```python
from build123d import *

# Parameters (mm, degrees)
EXTRUDE_1_DEPTH = 1
EXTRUDE_2_DEPTH = 1
EXTRUDE_3_REACH = 17
SKETCH_3_R      = 2.5


with BuildPart() as part:
    # 草图1 → 凸台-拉伸1 (new body)
    with BuildSketch(Plane(origin=(0, 0, 0), x_dir=(1, 0, 0), z_dir=(0, 1, 0))):
        with BuildLine():
            Line((-7, 15), (7, 15))
            ThreePointArc((7, 15), (7.707106781, 14.707106781), (8, 14))
            Line((8, 14), (8, -14))
            ThreePointArc((8, -14), (7.707106781, -14.707106781), (7, -15))
            Line((7, -15), (-7, -15))
            ThreePointArc((-7, -15), (-7.707106781, -14.707106781), (-8, -14))
            Line((-8, -14), (-8, 14))
            ThreePointArc((-8, 14), (-7.707106781, 14.707106781), (-7, 15))
        make_face()
    extrude(amount=EXTRUDE_1_DEPTH)

    # 草图2 → 凸台-拉伸2 (add)
    with BuildSketch(Plane.ZY.offset(8)):
        with BuildLine():
            Line((14, 1), (3.844755362, 32.532743309))
            ThreePointArc((3.844755362, 32.532743309), (-1.048573514, 35.998202631), (-5.749110975, 32.275431702))
            Line((-5.749110975, 32.275431702), (-14, 1))
            Line((-14, 1), (14, 1))
        make_face()
    extrude_2 = extrude(amount=-EXTRUDE_2_DEPTH)

    # 镜向1: 凸台-拉伸2 across plane
    add(extrude_2.mirror(Plane(origin=(0, 0, 0), x_dir=(0, 0, 1), z_dir=(1, 0, 0))))

    # 草图3 → 凸台-拉伸3 (add, up to next)
    with BuildSketch(Plane(origin=(-7, 0, 0), x_dir=(0, 0, -1), z_dir=(1, 0, 0)), mode=Mode.PRIVATE) as extrude_3_sk1:
        with Locations((0.914519578, 31)):
            Circle(SKETCH_3_R)
    extrude_3_tool1 = extrude(extrude_3_sk1.sketch, amount=EXTRUDE_3_REACH, mode=Mode.PRIVATE) - part.part
    add(extrude_3_tool1.solids().sort_by_distance((-7, 31, -0.91452))[0])


solid = part.part
```
The model under review builds one solid part; all positions refer to its coordinate system, in mm. A direction names the side the tool comes from. Give positions to 0.01 mm unless a question says otherwise; leave off trailing zeros. Write each loop counter-clockwise with the first axis right and the second up, starting at its lowest first coordinate (ties: lowest second). Pieces come first, ordered by that corner, then holes. Notation, with made-up numbers: M 12,70.25 L 45,70.25 A17 cw 45,93.25 Z; hole C 14,-18 d1. An arc over 180 degrees is marked long. Answer in a Markdown table with one row per item.
Item 1: For line 1 along X through (y, z) = (30, -4.5); line 2 along Y through (x, z) = (-6.25, 8.75); line 3 along Y through (x, z) = (-6.25, -3), list the stretches that pass through material, from the lowest coordinate up.
Check sheet entries:
| item | result |
|---|---|
| line 1 | -8 to -7, 7 to 8 |
| line 2 | 0 to 1 |
| line 3 | 0 to 1, 29.62 to 32.38 |
Item 2: Tool access review of faces 1 (the face through (7.507, 16.857, -9.817)), 2 (the face through (-0.098, 33.108, -2.259)): name each direction out of +Z, -Z, +X, -X, +Y, -Y from which nothing blocks a thin tool from reaching the whole face with its end or side.
Check sheet entries:
| item | result |
|---|---|
| face 1 | -Z, +X, -X, +Y |
| face 2 | none |
Item 3: Add section C-C on z = 6.5. Give the boundary of the cut face in (x, y).
Check sheet entries:
| item | result |
|---|---|
| outline | M -8,0 L 8,0 L 8,24.29 L 7,24.29 L 7,1 L -7,1 L -7,24.29 L -8,24.29 Z |
Item 4: Draft analysis for pull direction Y (two halves, no side actions). For faces 3 (the face through (-7.51, 16.55, 8.99)), 4 (the face through (-7, 15, 0)), 5 (the face through (-8, 14, 0)), state which applies: +Y half, -Y half, draft (parallel to the pull), parting line (faces both ways), or undercut.
Check sheet entries:
| item | result |
|---|---|
| face 3 | +Y half |
| face 4 | undercut |
| face 5 | draft |
Item 5: Add section D-D on y = 31. Give the boundary of the cut face in (x, z), plus the area to 3 significant figures.
Check sheet entries:
| item | result |
|---|---|
| outline | M -8,-6.09 L -7,-6.09 L -7,-3.41 L 7,-3.41 L 7,-6.09 L 8,-6.09 L 8,4.34 L 7,4.34 L 7,1.59 L -7,1.59 L -7,4.34 L -8,4.34 Z |
| area | 90.8 mm2 |
Item 6: For P1, Ø6, axis at x = 5, z = 3, coming from the +Y side; P2, Ø2, axis at x = 6.5, y = 29, coming from the -Z side; P3, Ø8, axis at x = 0.5, z = -1.5, coming from the +Y side, all flat-tipped, find the tip position at first contact; note any pin that passes through.
Check sheet entries:
| item | result |
|---|---|
| P1 | y = 35.71 |
| P2 | z = -6.84 |
| P3 | y = 33.5 |
Item 7: Add section B-B on y = 8. Give the boundary of the cut face in (x, z), plus the area to 3 significant figures.
Check sheet entries:
| item | result |
|---|---|
| outline | M -8,-12.15 L -7,-12.15 L -7,11.75 L -8,11.75 Z; M 7,-12.15 L 8,-12.15 L 8,11.75 L 7,11.75 Z |
| area | 47.8 mm2 |
Item 8: Add section A-A on x = -2.5. Give the boundary of the cut face in (y, z).
Check sheet entries:
| item | result |
|---|---|
| outline | M 0,-15 L 1,-15 L 1,15 L 0,15 Z; C 31,-0.91 d5 |
